The model under review builds one solid part; all positions refer to its coordinate system, in mm. Round coordinates to 2 decimals unless told otherwise and drop trailing zeros. Write each loop counter-clockwise with the first axis right and the second up, starting at its lowest first coordinate (ties: lowest second). Pieces come first, ordered by that corner, then holes.
Item 1: Add section A-A (z = 2.8). Give the boundary of the cut face in (x, y), plus the area to 4 significant figures.
Item 2: Clearance check with a flat-ended pin moving along its axis: pin 1 Ø1.2 at (x, z) = (0, 3) entering from +Y. State where the tip first meets the part, or that it passes through.
Item 3: To check wall thickness, follow L1, parallel to X at y = 24, z = 0.85; L2, parallel to Y at x = -5.5, z = 1.3. State the ranges of each line that lie inside material, in increasing order.
Item 4: Add section B-B (x = 96). Give the boundary of the cut face in (y, z).
Autodesk Inventor part; units mm, degrees
ref_plane "YZ Plane" through (0, 0, 0) normal (1, 0, 0) x (0, 1, 0)
ref_plane "XZ Plane" through (0, 0, 0) normal (0, 1, 0) x (-1, 0, 0)
ref_plane "XY Plane" through (0, 0, 0) normal (0, 0, 1) x (1, 0, 0)
sketch "Эскиз1" plane through (0, 0, 0) normal (0, 0, 1) x (1, 0, 0)
  line L0 (-142.5, 23) -> (142.5, 23)
  line L1 (142.5, 23) -> (142.5, -23)
  line L2 (142.5, -23) -> (-142.5, -23)
  line L3 (-142.5, -23) -> (-142.5, 23)
  line L4 (-142.5, 23) -> (142.5, -23) construction
  line L5 (142.5, 23) -> (-142.5, -23) construction
  point P0 (0, 0)
  dimension "d0" = 285
  dimension "d1" = 46
extrude "Выдавливание1" add sketch "Эскиз1" along normal blind 4
sketch "Эскиз2" plane through (-142.5, 23, 0) normal (0, 1, 0) x (1, 0, 0)
  line L0 (285, 0) -> (0, 0)
  line L1 (0, 0) -> (0, -4)
  line L2 (285, -4) -> (0, -4)
  line L3 (285, 0) -> (285, -4)
  line L4 (40, 0) -> (40, -4)
  line L5 (0, 0) -> (285, 0)
  line L6 (80, 0) -> (80, -4)
  line L7 (165, 0) -> (165, -4)
  line L8 (0, -4) -> (285, -4)
  line L9 (205, 0) -> (205, -4)
  line L10 (245, 0) -> (245, -4)
  line L11 (120, -4) -> (120, 0)
  point P0 (142.5, 0)
  point P1 (0, -2)
  point P2 (40, -2)
  point P3 (285, -2)
  point P4 (165, -2)
  point P5 (205, -2)
  point P6 (245, -2)
  point P7 (80, -2)
  point P8 (120, -2)
  dimension "d4" = 40
  dimension "d5" = 40
  dimension "d6" = 40
  dimension "d8" = 40
  dimension "d9" = 40
  dimension "d10" = 40
extrude "Выдавливание2" add sketch "Эскиз2" along normal blind 4 contours L3 L2 L10 L0 | L9 L2 L7 L0 | L11 L2 L6 L0 | L4 L2 L1 L0
properties part number "стенкаB"
Numbers:
1. outline: (-142.5, -23) - (142.5, -23) - (142.5, 27) - (102.5, 27) - (102.5, 23) - (62.5, 23) - (62.5, 27) - (22.5, 27) - (22.5, 23) - (-22.5, 23) - (-22.5, 27) - (-62.5, 27) - (-62.5, 23) - (-102.5, 23) - (-102.5, 27) - (-142.5, 27) - close
1. area: 13,750 mm2
2. pin 1: stops at y = 23
3. L1: x = -142.5 to -102.5, -62.5 to -22.5, 22.5 to 62.5, 102.5 to 142.5
3. L2: y = -23 to 23
4. outline: (-23, 0) - (23, 0) - (23, 4) - (-23, 4) - close
